Verification items for this drawing (mm, ordinates from the low corner). Coordinates: 2 decimals unless noted, no trailing zeros. Order: outer loops, then holes, each group sorted by start corner. A loop starts at its lowest first (then second) coordinate and runs counter-clockwise, first axis right, second up. Notation, with made-up numbers: M -23.75,-34 L 24.25,-34 A24 cw 24.25,-7 Z; hole C 57.5,9.25 d3. An arc over 180 degrees is marked long. Answer as a JSON object with one key per item and string values. Group by question number.
(1) Cross-section at C-C (z = 11). Enter the section's corners in (x, y).
(2) Material ranges on line 1 (X direction, y = 0.2, z = 20); line 2 (Z direction, x = 34, y = 1), recorded low to high.
(3) Gauge pin test, flat end, axial feed: pin 1 Ø1.5 at (x, z) = (51.5, 11) entering from -Y. Record the tip position at first contact, or that the pin passes through.
(4) Cross-section at A-A (x = 74). Enter the section's corners in (y, z).
(5) Cross-section at B-B (y = 0.8). Enter the section's corners in (x, z).
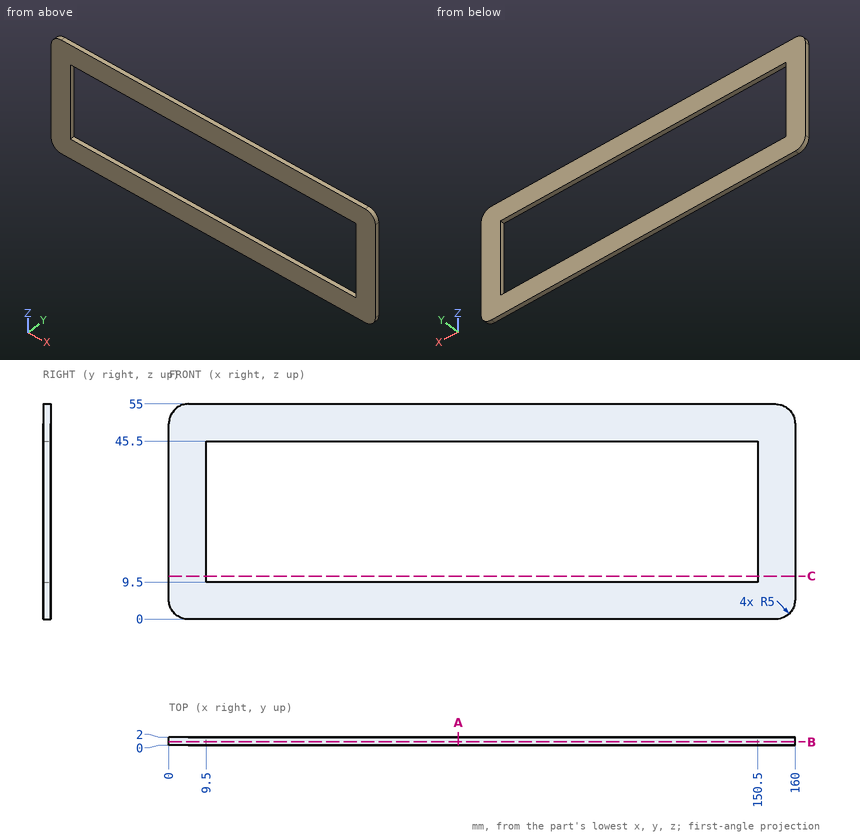
Taken from the geometry:
{
 "1": {"outline": "M 0,0 L 9.5,0 L 9.5,2 L 0,2 Z; M 150.5,0 L 160,0 L 160,2 L 150.5,2 Z"},
 "2": {"line 1": "x = 0 to 9.5, 150.5 to 160", "line 2": "z = 0 to 9.5, 45.5 to 55"},
 "3": {"pin 1": "passes through"},
 "4": {"outline": "M 0,0 L 2,0 L 2,9.5 L 0,9.5 Z; M 0,45.5 L 2,45.5 L 2,55 L 0,55 Z"},
 "5": {"outline": "M 0,5 A5 ccw 5,0 L 155,0 A5 ccw 160,5 L 160,50 A5 ccw 155,55 L 5,55 A5 ccw 0,50 Z; hole M 9.5,9.5 L 150.5,9.5 L 150.5,45.5 L 9.5,45.5 Z"}
}
